Geometry: see drawing. Coordinates: mm, zero at the bounding-box minimum. Coordinates: 2 decimals unless noted, no trailing zeros. Loops run counter-clockwise (first coordinate to the right, second up) from the corner with the lowest first, then second, coordinate; pieces in that order, holes last. Notation, with made-up numbers: (21.5, 51.25) - (52.5, 51.25) arc R28 ccw to (52.5, 78.25) - close; hole circle Ø3 at (73.5, 79). An arc over 180 degrees is marked (long way). Answer in a Markdown table with one row per item.
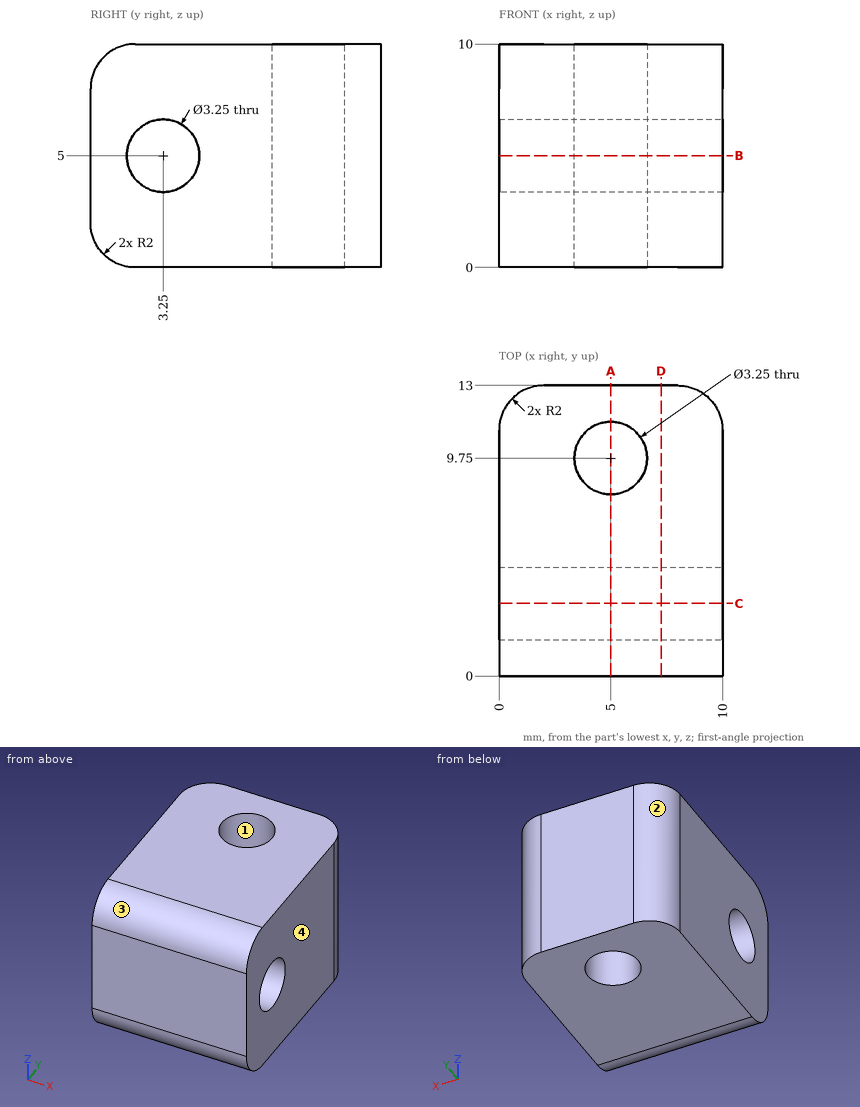
(1) Cut plane C-C on y = 3.25. Output: boundary loops of the cut face in (x, z) (3 decimals).
Verdict:
| item | result |
|---|---|
| outline | (0, 0) - (10, 0) - (10, 3.375) - (0, 3.375) - close; (0, 6.625) - (10, 6.625) - (10, 10) - (0, 10) - close |
(2) Pull-direction query (X, two-part tool) for the marked faces 1, 2, 3 and 4; classes: pulls with the +X half, pulls with the -X half, needs draft (parallel to the pull), parting line crosses it, or undercut.
Verdict:
| item | result |
|---|---|
| face 1 | undercut |
| face 2 | pulls with the -X half |
| face 3 | needs draft |
| face 4 | pulls with the +X half |
(3) Cut plane B-B on z = 5. Output: boundary loops of the cut face in (x, y) (3 decimals), then the cut area to 3 significant figures.
Verdict:
| item | result |
|---|---|
| outline | (0, 0) - (10, 0) - (10, 1.625) - (0, 1.625) - close; (0, 4.875) - (10, 4.875) - (10, 11) arc R2 ccw to (8, 13) - (2, 13) arc R2 ccw to (0, 11) - close; hole circle Ø3.25 at (5, 9.75) |
| area | 87.5 mm² |
(4) First-contact query: pin 1 Ø1.5 at (x, z) = (1, 7.5) entering from +Y. Flat tip, straight axial feed; report the tip coordinate or a pass-through.
Verdict:
| item | result |
|---|---|
| pin 1 | stops at y = 12.98 |
(5) Cut plane A-A on x = 5. Output: boundary loops of the cut face in (y, z) (3 decimals), then the cut area to 3 significant figures.
Verdict:
| item | result |
|---|---|
| outline | (0, 2) arc R2 ccw to (2, 0) - (8.125, 0) - (8.125, 10) - (2, 10) arc R2 ccw to (0, 8) - close; (11.375, 0) - (13, 0) - (13, 10) - (11.375, 10) - close; hole circle Ø3.25 at (3.25, 5) |
| area | 87.5 mm² |
(6) Cut plane D-D on x = 7.25. Output: boundary loops of the cut face in (y, z) (3 decimals), then the cut area to 3 significant figures.
Verdict:
| item | result |
|---|---|
| outline | (0, 2) arc R2 ccw to (2, 0) - (13, 0) - (13, 10) - (2, 10) arc R2 ccw to (0, 8) - close; hole circle Ø3.25 at (3.25, 5) |
| area | 120 mm² |
(7) Ray query, probe 1 along X at (y, z) = (9.75, 4) (3 decimals); probe 2 along Y at (x, z) = (5, 3) (3 decimals). Return the intervals inside material, ascending.
Verdict:
| item | result |
|---|---|
| probe 1 | x = 0 to 3.375, 6.625 to 10 |
| probe 2 | y = 0 to 8.125, 11.375 to 13 |
